Source: CAD feature listing. Evaluate the final solid. Frame: model axes, mm. A direction names the side the tool comes from. Round coordinates to 2 decimals unless told otherwise and drop trailing zeros. Write each loop counter-clockwise with the first axis right and the second up, starting at its lowest first coordinate (ties: lowest second). Pieces come first, ordered by that corner, then holes. Notation, with made-up numbers: M -12.5,-21.75 L -0.5,-21.75 A38 cw -0.5,16.25 Z; hole C -10.75,-13 d2. An arc over 180 degrees is marked long. Answer in a Markdown table with one row per item.
from build123d import *

# Parameters (mm, degrees)
SKETCH_1_R      = 4.5
SKETCH_1_R_2    = 2
SKETCH_1_R_3    = 1.25
EXTRUDE_2_DEPTH = 0.5
SKETCH_2_R      = 4.5
SKETCH_2_R_2    = 2
SKETCH_2_R_3    = 1.25
EXTRUDE_3_DEPTH = 4.5
SKETCH_3_R      = 15
SKETCH_3_R_2    = 1.25
EXTRUDE_4_DEPTH = 0.5


with BuildPart() as part:
    # 草图1 → 凸台-拉伸2 (new body)
    with BuildSketch(Plane(origin=(0, 0, 0), x_dir=(1, 0, 0), z_dir=(0, 1, 0))):
        with BuildLine():
            Line((-14.860465116, 23.546511628), (-14.860465116, -16.170631515))
            ThreePointArc((-14.860465116, -16.170631515), (-15.250692888, -18.107123188), (-16.360465116, -19.741345729))
            ThreePointArc((-16.360465116, -19.741345729), (-5.860465116, -45.453488372), (4.639534884, -19.741345729))
            ThreePointArc((4.639534884, -19.741345729), (3.529762655, -18.107123188), (3.139534884, -16.170631515))
            Line((3.139534884, -16.170631515), (3.139534884, 3.546511628))
            Line((3.139534884, 3.546511628), (3.139534884, 23.546511628))
            ThreePointArc((3.139534884, 23.546511628), (-5.860465116, 32.546511628), (-14.860465116, 23.546511628))
        make_face()
        with Locations(Location((-5.860465116, 23.546511628, 0), (0, 0, 270))):
            Circle(SKETCH_1_R, mode=Mode.SUBTRACT)
        with Locations(Location((-5.860465116, 3.546511628, 0), (0, 0, 270))):
            Circle(SKETCH_1_R_2, mode=Mode.SUBTRACT)
        with Locations(Location((-5.860465116, -30.453488372, 0), (0, 0, 270))):
            Circle(SKETCH_1_R, mode=Mode.SUBTRACT)
        with Locations(Location((-15.766516879, -29.085958307, 0), (0, 0, 270))):
            Circle(SKETCH_1_R_3, mode=Mode.SUBTRACT)
        with Locations(Location((-2.091755012, -39.716145882, 0), (0, 0, 270))):
            Circle(SKETCH_1_R_3, mode=Mode.SUBTRACT)
        with Locations(Location((0.276876542, -22.558360927, 0), (0, 0, 270))):
            Circle(SKETCH_1_R_3, mode=Mode.SUBTRACT)
    extrude(amount=EXTRUDE_2_DEPTH)

    # 草图2 → 凸台-拉伸3 (add)
    with BuildSketch(Plane(origin=(0, 0.5, 0), x_dir=(1, 0, 0), z_dir=(0, 1, 0))):
        with BuildLine():
            Line((-14.860465116, 23.546511628), (-14.860465116, -16.170631515))
            ThreePointArc((-14.860465116, -16.170631515), (-15.250692888, -18.107123188), (-16.360465116, -19.741345729))
            ThreePointArc((-16.360465116, -19.741345729), (-5.860465116, -45.453488372), (4.639534884, -19.741345729))
            ThreePointArc((4.639534884, -19.741345729), (3.529762655, -18.107123188), (3.139534884, -16.170631515))
            Line((3.139534884, -16.170631515), (3.139534884, 23.546511628))
            ThreePointArc((3.139534884, 23.546511628), (-5.860465116, 32.546511628), (-14.860465116, 23.546511628))
        make_face()
        with Locations(Location((-5.860465116, 23.546511628, 0), (0, 0, 270))):
            Circle(SKETCH_2_R, mode=Mode.SUBTRACT)
        with Locations(Location((-5.860465116, 3.546511628, 0), (0, 0, 270))):
            Circle(SKETCH_2_R_2, mode=Mode.SUBTRACT)
        with Locations(Location((-15.766516879, -29.085958307, 0), (0, 0, 270))):
            Circle(SKETCH_2_R_3, mode=Mode.SUBTRACT)
        with Locations(Location((-2.091755012, -39.716145882, 0), (0, 0, 270))):
            Circle(SKETCH_2_R_3, mode=Mode.SUBTRACT)
        with Locations(Location((0.276876542, -22.558360927, 0), (0, 0, 270))):
            Circle(SKETCH_2_R_3, mode=Mode.SUBTRACT)
    extrude(amount=EXTRUDE_3_DEPTH)

    # 草图3 → 凸台-拉伸4 (add)
    with BuildSketch(Plane(origin=(0, 5, 0), x_dir=(1, 0, 0), z_dir=(0, 1, 0))):
        with Locations(Location((-5.860465116, -30.453488372, 0), (0, 0, 45.572995999))):
            Circle(SKETCH_3_R)
        with Locations(Location((-15.766516879, -29.085958307, 0), (0, 0, 270))):
            Circle(SKETCH_3_R_2, mode=Mode.SUBTRACT)
        with Locations(Location((0.276876542, -22.558360927, 0), (0, 0, 270))):
            Circle(SKETCH_3_R_2, mode=Mode.SUBTRACT)
        with Locations(Location((-2.091755012, -39.716145882, 0), (0, 0, 270))):
            Circle(SKETCH_3_R_2, mode=Mode.SUBTRACT)
    extrude(amount=EXTRUDE_4_DEPTH)


solid = part.part
Q1. Section C-C (x = -12). Return loops of the section in (y, z), and give its area (3 significant figures).
Solutions:
| item | result |
|---|---|
| outline | M 0,-30.13 L 5,-30.13 L 5,16.77 L 5.5,16.77 L 5.5,44.14 L 0,44.14 Z |
| area | 385 mm2 |
Q2. Access query for faces 1 (the flat face through (3.14, 2, -3)), 2 (the flat face through (-6, 0.5, 30)), 3 (the cylindrical face through (-7.635, 2.465, -2.624)). Directions: +Z, -Z, +X, -X, +Y, -Y. A direction counts if a zero-diameter tool reaches every point of the face in a straight line with its end or side. Return the directions, or none.
Solutions:
| item | result |
|---|---|
| face 1 | -Z, +X, +Y, -Y |
| face 2 | -Y |
| face 3 | +Y, -Y |
Q3. Section A-A (y = 1.7). Return loops of the section in (x, z).
Solutions:
| item | result |
|---|---|
| outline | M -16.36,19.74 A5 cw -14.86,16.17 L -14.86,-23.55 A9 ccw 3.14,-23.55 L 3.14,16.17 A5 cw 4.64,19.74 A15 ccw long Z; hole C -15.77,29.09 d2.5; hole C -5.86,-23.55 d9; hole C -5.86,-3.55 d4; hole C -2.09,39.72 d2.5; hole C 0.28,22.56 d2.5 |
Q4. Material intervals for probe 1 along Z at (x, y) = (-6, 3.65); probe 2 along Z at (x, y) = (-5.5, 2.5); probe 3 along X at (y, z) = (1.8, -1.5), sorted ascending.
Solutions:
| item | result |
|---|---|
| probe 1 | z = -32.55 to -28.04, -19.05 to -5.54, -1.55 to 45.45 |
| probe 2 | z = -32.54 to -28.03, -19.06 to -5.51, -1.58 to 45.45 |
| probe 3 | x = -14.86 to 3.14 |
Q5. Contact query for flat-ended pins moving along their axis: pin 1 Ø1.5 at (x, y) = (-14.5, 3.5) entering from +Z; pin 2 Ø2.5 at (y, z) = (2, -3.5) entering from -X; pin 3 Ø2 at (x, y) = (-17.5, 1) entering from +Z; pin 4 Ø8 at (x, z) = (-5.86, -23.55) entering from +Y. Output: stop coordinate, or through.
Solutions:
| item | result |
|---|---|
| pin 1 | stops at z = 43.21 |
| pin 2 | stops at x = -14.86 |
| pin 3 | stops at z = 41.03 |
| pin 4 | passes through |
Q6. Section D-D (z = 25). Return loops of the section in (x, y), and give its area (3 significant figures).
Solutions:
| item | result |
|---|---|
| outline | M -19.83,0 L 8.11,0 L 8.11,5.5 L -19.83,5.5 Z |
| area | 154 mm2 |
Q7. Pull-direction query (X, two-part tool) for faces 4 (the flat face through (-14.86, 2, -4)), 5 (the cylindrical face through (-7.58, 0.25, 34.61)), 6 (the cylindrical face through (3.54, 2.46, 18.13)); classes: pulls with the +X half, pulls with the -X half, needs draft (parallel to the pull), parting line crosses it, or undercut.
Solutions:
| item | result |
|---|---|
| face 4 | pulls with the -X half |
| face 5 | undercut |
| face 6 | pulls with the +X half |
Q8. Section B-B (z = 11). Return loops of the section in (x, y), and give its area (3 significant figures).
Solutions:
| item | result |
|---|---|
| outline | M -14.86,0 L 3.14,0 L 3.14,5 L -14.86,5 Z |
| area | 90.0 mm2 |
